The listing builds one solid part. Answer for the finished solid, in the listing's coordinates (mm). Face numbers are marked on the shaded views. A direction names the side the tool comes from. Coordinates: 2 decimals unless noted, no trailing zeros. Order: outer loops, then holes, each group sorted by start corner. A loop starts at its lowest first (then second) coordinate and runs counter-clockwise, first axis right, second up.
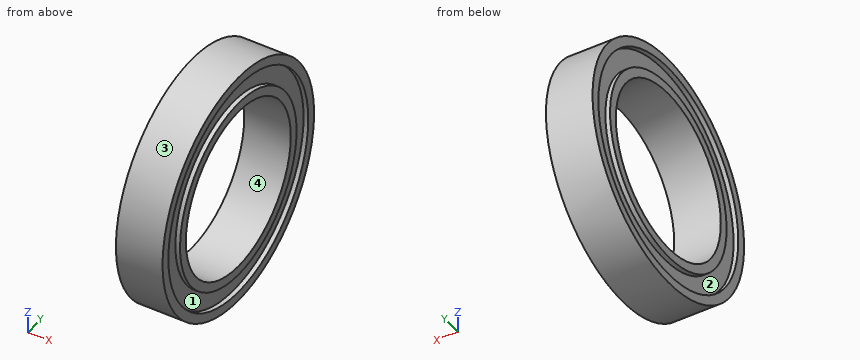
```python
from build123d import *

# Parameters (mm, degrees)
SKETCH2_R           = 13
BOSS_EXTRUDE1_DEPTH = 2.5
SKETCH3_R           = 9
CUT_EXTRUDE1_DEPTH  = 6
SKETCH4_R           = 12
SKETCH4_R_2         = 11
SKETCH4_R_3         = 10
CUT_EXTRUDE2_DEPTH  = 0.5


with BuildPart() as part:
    # Sketch2 → Boss-Extrude1 (new, symmetric)
    with BuildSketch(Plane(origin=(0, 0, 0), x_dir=(0, 0, -1), z_dir=(1, 0, 0))):
        Circle(SKETCH2_R)
    extrude(amount=BOSS_EXTRUDE1_DEPTH, both=True)

    # Sketch3 → Cut-Extrude1 (cut)
    with BuildSketch(Plane(origin=(2.5, 0, 0), x_dir=(0, 0, -1), z_dir=(1, 0, 0))):
        Circle(SKETCH3_R)
    extrude(amount=-CUT_EXTRUDE1_DEPTH, mode=Mode.SUBTRACT)

    # Sketch4 → Cut-Extrude2 (cut)
    with BuildSketch(Plane(origin=(2.5, 0, 0), x_dir=(0, 0, -1), z_dir=(1, 0, 0))):
        Circle(SKETCH4_R)
        Circle(SKETCH4_R_2, mode=Mode.SUBTRACT)
        Circle(SKETCH4_R_2)
        Circle(SKETCH4_R_3, mode=Mode.SUBTRACT)
    cut_extrude2 = extrude(amount=-CUT_EXTRUDE2_DEPTH, mode=Mode.SUBTRACT)

    # Mirror1: Cut-Extrude2 across plane
    add(cut_extrude2.mirror(Plane(origin=(0, 0, 0), x_dir=(0, 0, 1), z_dir=(1, 0, 0))), mode=Mode.SUBTRACT)


solid = part.part
```
(1) Find section C-C (x = 1.5). Write down the section's boundary in (y, z).
(2) Consider line 1 (Y direction, x = -2.3, z = 0); line 2 (Y direction, x = -0.05, z = 0). Determine where each line is inside the solid, lowest interval first.
(3) For the marked faces 1 and 2, determine the directions among +Z, -Z, +X, -X, +Y, -Y from which every point of the face is accessible in a straight line to the end or side of a thin tool.
(4) The mould has two halves that part along Z. Classify the marked faces 3 and 4: released by +Z, released by -Z, zero draft, split by the parting line, or undercut.
(5) Each of these flat-tipped pins is pushed along its axis until it touches: pin 1 Ø7 at (y, z) = (3.5, 3) entering from +X; pin 2 Ø1.5 at (x, z) = (1, 2.5) entering from -Y; pin 3 Ø1.5 at (y, z) = (-8, -4) entering from -X; pin 4 Ø1.5 at (y, z) = (-10, -4.5) entering from +X. Where does it stop, or does it pass through?
(6) Find section A-A (y = 0). Write down the section's boundary in (x, z), and give its area (3 significant figures).
Findings below:
1. outline: circle Ø26 at (0, 0); hole circle Ø18 at (0, 0)
2. line 1: y = -13 to -12, -10 to -9, 9 to 10, 12 to 13
2. line 2: y = -13 to -9, 9 to 13
3. face 1: +X
3. face 2: -X
4. face 3: split by the parting line
4. face 4: undercut
5. pin 1: passes through
5. pin 2: stops at y = -12.88
5. pin 3: stops at x = -2.5
5. pin 4: stops at x = 2
6. outline: (-2.5, -13) - (2.5, -13) - (2.5, -12) - (2, -12) - (2, -10) - (2.5, -10) - (2.5, -9) - (-2.5, -9) - (-2.5, -10) - (-2, -10) - (-2, -12) - (-2.5, -12) - close; (-2.5, 9) - (2.5, 9) - (2.5, 10) - (2, 10) - (2, 12) - (2.5, 12) - (2.5, 13) - (-2.5, 13) - (-2.5, 12) - (-2, 12) - (-2, 10) - (-2.5, 10) - close
6. area: 36.0 mm2
